Autodesk Inventor part; units mm, degrees
ref_plane "YZ Plane" through (0, 0, 0) normal (1, 0, 0) x (0, 1, 0)
ref_plane "XZ Plane" through (0, 0, 0) normal (0, 1, 0) x (-1, 0, 0)
ref_plane "XY Plane" through (0, 0, 0) normal (0, 0, 1) x (1, 0, 0)
sketch "Sketch1" plane through (0, 0, 0) normal (0, 0, 1) x (1, 0, 0)
  line L0 (142.5, 18) -> (-142.5, 18)
  line L1 (-142.5, 18) -> (-142.5, -18)
  line L2 (-142.5, -18) -> (142.5, -18)
  line L3 (142.5, -18) -> (142.5, 18)
  line L4 (142.5, 18) -> (-142.5, -18) construction
  line L5 (-142.5, 18) -> (142.5, -18) construction
  line L6 (-142.5, 18) -> (142.5, 18)
  line L7 (142.5, 18) -> (142.5, 8)
  line L8 (142.5, 8) -> (-142.5, 8)
  line L9 (-142.5, 8) -> (-142.5, 18)
  point P0 (0, 0)
  point P1 (142.5, 13)
  dimension "d0" = 285
  dimension "d1" = 36
  dimension "d4" = 5
extrude "Extrusion1" add sketch "Sketch1" along normal blind 10
sketch "Sketch4" plane through (0, 0, 10) normal (0, 0, 1) x (1, 0, 0)
  line L0 (-142.5, 18) -> (-142.5, -18)
  line L1 (-142.5, 18) -> (142.5, 18)
  line L2 (142.5, 18) -> (142.5, 13)
  line L3 (142.5, 13) -> (-142.5, 13)
  line L4 (-142.5, 13) -> (-142.5, 18)
  point P0 (0, 0)
  dimension "d5" = 285
  dimension "d6" = 5
extrude "Extrusion2" add sketch "Sketch4" along normal blind 15
sketch "Sketch5" plane through (0, 0, 10) normal (0, 0, 1) x (1, 0, 0)
  line L0 (-142.5, 18) -> (-142.5, -18)
  line L1 (-142.5, 7) -> (142.5, 7)
  line L2 (142.5, 7) -> (142.5, 2)
  line L3 (142.5, 2) -> (-142.5, 2)
  line L4 (-142.5, 2) -> (-142.5, 7)
  line L5 (142.5, 13) -> (-142.5, 13)
  point P0 (0, 0)
  dimension "d9" = 285
  dimension "d10" = 5
  dimension "d47" = 11
extrude "Extrusion3" add sketch "Sketch5" along normal blind 15
fillet "Fillet1" radius 7.5 1 edges at (0, 2, 10)
sketch "Sketch11" plane through (0, 0, 0) normal (0, 0, -1) x (-1, 0, 0)
  circle A0 centre (-69.4481, -8.5) radius 2.5
  circle A1 centre (-69.4481, -8.5) radius 2.1
  circle A2 centre (0, -8.5) radius 2.5
  circle A3 centre (0, -8.5) radius 2.1
  circle A4 centre (70, -8.5) radius 2.5
  circle A5 centre (70, -8.5) radius 2.1
  point P0 (0, 0)
  dimension "d52" = 4.2
  dimension "d53" = 4.2
  dimension "d54" = 4.2
extrude "Extrusion4" cut sketch "Sketch11" against normal through all contours A1 | A2 | A3 | A4 | A5
equation "\"d53\" = d52"
equation "\"d54\" = d52"
properties part number "cheeseboard mounts v02"
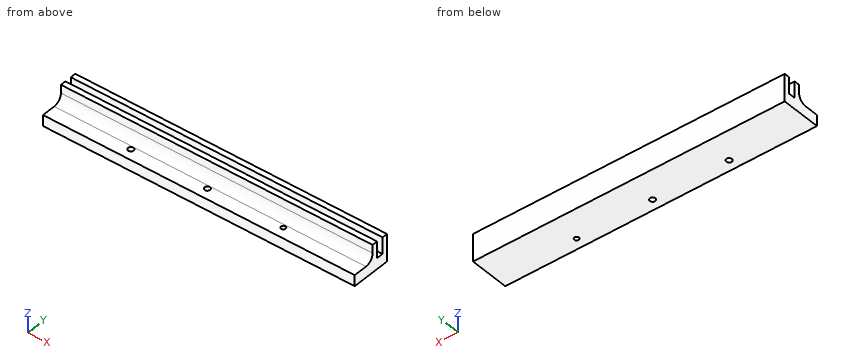
Input: part model. Units: mm. Frame: model coordinates. Coordinates: 2 decimals unless noted, no trailing zeros. Write each loop counter-clockwise with the first axis right and the second up, starting at its lowest first coordinate (ties: lowest second). Pieces come first, ordered by that corner, then holes. Notation, with made-up numbers: (59.25, -32.5) -> (84.25, -32.5) arc R18 cw to (84.25, -12.5) -> close; hole circle Ø2 at (41, 64). An arc over 180 degrees is marked (long way). Write each question's results on one line, items separated by ' | '.
Item 1: Section query B-B on x = 0. Return loops of the section in (y, z).
Conclusion:
outline: (-18, 0) -> (-11, 0) -> (-11, 10) -> (-18, 10) -> close; (-6, 0) -> (18, 0) -> (18, 25) -> (13, 25) -> (13, 10) -> (7, 10) -> (7, 25) -> (2, 25) -> (2, 17.5) arc R7.5 cw to (-5.5, 10) -> (-6, 10) -> close
Item 2: Material intervals for probe 1 along Y at (x, z) = (57.5, 21.5); probe 2 along Y at (x, z) = (-70, 6.25); probe 3 along Z at (x, y) = (58, -6), sorted ascending.
Conclusion:
probe 1: y = 2 to 7, 13 to 18 | probe 2: y = -18 to -11, -6 to 18 | probe 3: z = 0 to 10
Item 3: Section query A-A on z = 13. Return loops of the section in (x, y).
Conclusion:
outline: (-142.5, 0.5) -> (142.5, 0.5) -> (142.5, 7) -> (-142.5, 7) -> close; (-142.5, 13) -> (142.5, 13) -> (142.5, 18) -> (-142.5, 18) -> close
Item 4: Pin query (flat end, axial travel): pin 1 Ø6.5 at (x, y) = (63.5, 10) entering from +Z; pin 2 Ø2 at (x, y) = (-8.5, 9.5) entering from +Z; pin 3 Ø7.5 at (x, z) = (-46, 17.5) entering from -Y; pin 4 Ø14 at (x, y) = (27, -11.5) entering from +Z. Return the tip coordinate at first contact, or that it passes through.
Conclusion:
pin 1: stops at z = 25 | pin 2: stops at z = 10 | pin 3: stops at y = 1 | pin 4: stops at z = 10.07
Item 5: Section query C-C on x = -57. Return loops of the section in (y, z), plus the area to 3 significant figures.
Conclusion:
outline: (-18, 0) -> (18, 0) -> (18, 25) -> (13, 25) -> (13, 10) -> (7, 10) -> (7, 25) -> (2, 25) -> (2, 17.5) arc R7.5 cw to (-5.5, 10) -> (-18, 10) -> close | area: 522 mm^2
